from build123d import *

# Parameters (mm, degrees)
BOSS_EXTRUDE1_DEPTH = 3.175
SKETCH3_W           = 3.175
SKETCH3_H           = 14.8
CUT_EXTRUDE1_DEPTH  = 4.1750001
SKETCH4_W           = 9.8
SKETCH4_H           = 3.175
SKETCH4_W_2         = 15
CUT_EXTRUDE2_DEPTH  = 3.175
CUT_EXTRUDE3_DEPTH  = 4.1750001


with BuildPart() as part:
    # Sketch1 → Boss-Extrude1 (new body)
    with BuildSketch(Plane.XY):
        with BuildLine():
            Line((0, 0), (65, 0))
            Line((65, 0), (76.490666647, 9.641814145))
            add(Edge.make_bspline(
                [(76.490666647, 9.641814145), (35.667607653, 68.4177286), (-16.08044376, 52.596761578)],
                knots=[0, 0, 0, 1, 1, 1], degree=2))
            Line((-16.08044376, 52.596761578), (0, 0))
        make_face()
    extrude(amount=BOSS_EXTRUDE1_DEPTH)

    # Sketch3 → Cut-Extrude1 (cut, through all)
    with BuildSketch(Plane(origin=(0, 0, 0), x_dir=(-1, 0, 0), z_dir=(0, 0, -1))):
        with Locations((-40.601722956, 31.627041635)):
            Rectangle(SKETCH3_W, SKETCH3_H)
        Polygon((-24.165936956, 40.667408524), (-21.242219909, 50.230456083), (-18.205952308, 49.302175921), (-21.129669356, 39.739128361), align=None)
        Polygon((-24.111860744, 29.984819851), (-27.148128344, 30.913100013), (-30.01337105, 21.541313405), (-26.97710345, 20.613033242), align=None)
        Polygon((-26.048823288, 23.649300842), (-26.97710345, 20.613033242), (-17.414055891, 17.689316195), (-16.485775728, 20.725583795), align=None)
        Polygon((-1.470619079, 44.185671088), (1.453097968, 53.748718648), (4.489365568, 52.820438485), (1.565648521, 43.257390926), align=None)
        Polygon((-10.241770221, 15.496528409), (-7.205502621, 14.568248247), (-6.277222458, 17.604515847), (-4.340259914, 23.940034855), (-7.376527515, 24.868315018), align=None)
        Polygon((-7.205502621, 14.568248247), (3.457295408, 11.308303739), (4.385575571, 14.344571339), (-6.277222458, 17.604515847), align=None)
    extrude(amount=-CUT_EXTRUDE1_DEPTH, mode=Mode.SUBTRACT)

    # Sketch4 → Cut-Extrude2 (cut)
    with BuildSketch(Plane(origin=(0, 0, 0), x_dir=(-1, 0, 0), z_dir=(0, 0, -1))):
        with Locations((-14.9, 1.5875)):
            Rectangle(SKETCH4_W, SKETCH4_H)
        with Locations((-47.5, 1.5875)):
            Rectangle(SKETCH4_W_2, SKETCH4_H)
        Polygon((13.01054086, 42.55556164), (9.97427326, 43.483841803), (1.349307971, 15.272851502), (4.385575571, 14.344571339), align=None)
    extrude(amount=-CUT_EXTRUDE2_DEPTH, mode=Mode.SUBTRACT)

    # Sketch5 → Cut-Extrude3 (cut, through all)
    with BuildSketch(Plane.XY.offset(3.175)):
        Polygon((11.804307663, 9.030936103), (53.371240129, 21.739222692), (64.034758718, 9.030936103), align=None)
        Polygon((5.306009056, 43.811965436), (10.721102585, 26.099992585), (20.789996423, 29.178362359), (15.374902893, 46.890335211), align=None)
    extrude(amount=-CUT_EXTRUDE3_DEPTH, mode=Mode.SUBTRACT)


solid = part.part
Build history of the part. All positions in model axes, mm. A direction names the side the tool comes from. Coordinates: 2 decimals unless noted, no trailing zeros. Write each loop counter-clockwise with the first axis right and the second up, starting at its lowest first coordinate (ties: lowest second). Pieces come first, ordered by that corner, then holes.
(1) Pin check, flat tips, straight feed: pin 1 Ø8 at (x, y) = (23.5, 44.5) entering from -Z; pin 2 Ø1.6 at (x, z) = (16, 1.5) entering from -Y (3 decimals); pin 3 Ø1.6 at (y, z) = (1, 2) entering from -X; pin 4 Ø1.6 at (y, z) = (32, 2) entering from -X. Stop position of each tip, or through.
(2) Cut at A-A on z = 2.35. State how many separate pieces and enclosed holes the cut face has, and give its area (3 significant figures).
(3) 3-axis set-ups, long thin cutter, end or side, ignore diameter. For faces 4 (the flat face through (70.66, 4.75, 1.57)), 5 (the flat face through (5.32, 20.73, 1.57)), 6 (the flat face through (40, 2, 2)): which of +Z, -Z, +X, -X, +Y, -Y reach the whole face in a straight line?
(4) Cut at C-C on y = 5.5. List the corners of the cut face in (x, z) (3 decimals), and give its area (3 significant figures).
(5) Mould opens along Y. For faces 1 (the flat face through (55, 2, 2)), 2 (the flat face through (-11.514, 43.013, 1.565)), 3 (the flat face through (10.411, 45.373, 1.61)) say: pulls with the +Y half, pulls with the -Y half, needs draft (parallel to the pull), parting line crosses it, or undercut.
(6) Drill centre lines: line 1 (X direction, y = 33.5, z = 0.45); line 2 (X direction, y = 29.5, z = 0.35) (3 decimals); line 3 (X direction, y = 33, z = 2.1). Where is each one in solid material? Low to high.
Working result:
1. pin 1: stops at z = 0
1. pin 2: stops at y = 3.175
1. pin 3: stops at x = -0.55
1. pin 4: stops at x = -6.71
2. separate pieces: 1
2. enclosed holes: 6
2. area: 2,690 mm2
3. face 4: +Z, -Z, +X, -Y
3. face 5: +Z, -Z
3. face 6: +Z, -Z, -Y
4. outline: (-1.682, 0) - (71.555, 0) - (71.555, 3.175) - (-1.682, 3.175) - close
4. area: 233 mm2
5. face 1: needs draft
5. face 2: pulls with the -Y half
5. face 3: undercut
6. line 1: x = -6.92 to 8.46, 19.47 to 39.01, 42.19 to 56.33
6. line 2: x = -5.699 to 9.682, 20.692 to 24.26, 27.58 to 39.014, 42.189 to 60.375
6. line 3: x = -6.77 to 8.61, 19.62 to 39.01, 42.19 to 56.85
